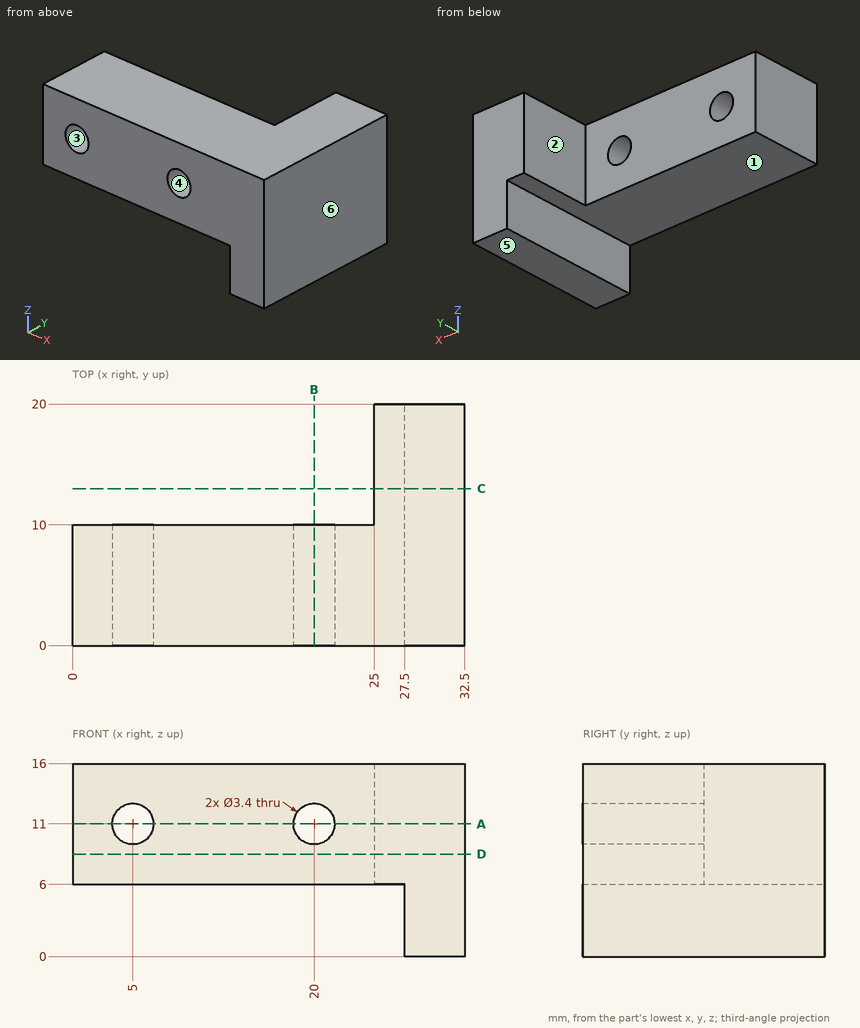
Source: three-view drawing plus pictorial views. Frame: mm from the lowest corner of the part. A direction names the side the tool comes from. Coordinates: 2 decimals unless noted, no trailing zeros. Write each loop counter-clockwise with the first axis right and the second up, starting at its lowest first coordinate (ties: lowest second). Pieces come first, ordered by that corner, then holes. Notation, with made-up numbers: (-17, 33.5) - (-5, 33.5) arc R22 ccw to (-5, 40.5) - close; hole circle Ø3 at (35, 31.5). An arc over 180 degrees is marked (long way). Answer as a JSON object with one key per item and string values.
Q1. First-contact query: pin 1 Ø6 at (x, y) = (19, 9.5) entering from -Z; pin 2 Ø3 at (y, z) = (12, 3.5) entering from -X; pin 3 Ø4.5 at (x, z) = (5, 11) entering from +Y. Flat tips, straight axial feed; report the tip coordinate or a pass-through.
Ans:
{"pin 1": "stops at z = 6", "pin 2": "stops at x = 27.5", "pin 3": "stops at y = 10"}
Q2. Material intervals for line 1 (X direction, y = 7.25, z = 11); line 2 (X direction, y = 2.25, z = 10.5); line 3 (Y direction, x = 8.5, z = 11.5), sorted ascending. Write a range as [from, to].
Ans:
{"line 1": "x = [0, 3.3], [6.7, 18.3], [21.7, 32.5]", "line 2": "x = [0, 3.38], [6.62, 18.38], [21.62, 32.5]", "line 3": "y = [0, 10]"}
Q3. Section query A-A, the plane z = 11. Output: boundary loops of the cut face in (x, y).
Ans:
{"outline": "(0, 0) - (3.3, 0) - (3.3, 10) - (0, 10) - close; (6.7, 0) - (18.3, 0) - (18.3, 10) - (6.7, 10) - close; (21.7, 0) - (32.5, 0) - (32.5, 20) - (25, 20) - (25, 10) - (21.7, 10) - close"}
Q4. Section query B-B, the plane x = 20. Output: boundary loops of the cut face in (y, z), plus the area to 3 significant figures.
Ans:
{"outline": "(0, 6) - (10, 6) - (10, 9.3) - (0, 9.3) - close; (0, 12.7) - (10, 12.7) - (10, 16) - (0, 16) - close", "area": "66.0 mm2"}
Q5. Section query D-D, the plane z = 8.5. Output: boundary loops of the cut face in (x, y), plus the area to 3 significant figures.
Ans:
{"outline": "(0, 0) - (32.5, 0) - (32.5, 20) - (25, 20) - (25, 10) - (0, 10) - close", "area": "400 mm2"}
Q6. Draft query along Z for the marked faces 4, 5 and 6. Return one class per face: released by +Z, released by -Z, zero draft, split by the parting line, or undercut.
Ans:
{"face 4": "undercut", "face 5": "released by -Z", "face 6": "zero draft"}
Q7. Set-up query: the marked faces 1, 2 and 3. Return all of +Z, -Z, +X, -X, +Y, -Y with unobstructed straight access to the full face (end or side cutting, diameter ignored); none if empty.
Ans:
{"face 1": "-Z, -X, +Y, -Y", "face 2": "+Z, -Z, -X, +Y", "face 3": "+Y, -Y"}
Q8. Section query C-C, the plane y = 13. Output: boundary loops of the cut face in (x, z), plus the area to 3 significant figures.
Ans:
{"outline": "(25, 6) - (27.5, 6) - (27.5, 0) - (32.5, 0) - (32.5, 16) - (25, 16) - close", "area": "105 mm2"}
